Source: CAD feature listing. Evaluate the final solid. Frame: model axes, mm. Give positions to 0.01 mm unless a question says otherwise; leave off trailing zeros. Loops run counter-clockwise (first coordinate to the right, second up) from the corner with the lowest first, then second, coordinate; pieces in that order, holes last. Notation, with made-up numbers: (24.25, -12.5) - (43.25, -12.5) arc R24 ccw to (43.25, 19.5) - close; hole circle Ø7 at (66, 75). An arc over 180 degrees is marked (long way). Write each question's results on one line, items separated by ' | '. Start each with the question number.
(1) Cut plane B-B on y = 13.5. Return the cut outline in (x, z), then the cut area to 3 significant figures.
(2) Material intervals for line 1 along Z through (x, y) = (0.05, 14.75); line 2 along Y through (x, z) = (1.35, -2); line 3 along X through (y, z) = (1.5, -0.5), sorted ascending. Write a range as [from, to].
(3) Pull-direction query (X, two-part tool) for faces 1 (the flat face through (0, 21.7, 0)), 2 (the cylindrical face through (-1.5, 10.01, -0.07)), 3 (the flat face through (0, 0, 0)); classes: pulls with the +X half, pulls with the -X half, needs draft (parallel to the pull), parting line crosses it, or undercut.
(4) Contact query for flat-ended pins moving along their axis: pin 1 (2 mm diameter, centred on y = 15.5, z = 0, fed in from +X); pin 2 (2 mm diameter, centred on x = 1, y = 13.5, fed in from -Z). Output: stop coordinate, or through.
from build123d import *

# Parameters (mm, degrees)
SKETCH1_R           = 1.5
BOSS_EXTRUDE1_DEPTH = 22
SKETCH2_R           = 2.6
BOSS_EXTRUDE2_DEPTH = 1.7
BOSS_EXTRUDE2_TAPER = 32
SKETCH3_W           = 0.5
SKETCH3_H           = 1.758378485
SKETCH3_H_2         = 1.741621515
SKETCH3_W_2         = 1.734727157
SKETCH3_H_3         = 0.5
SKETCH3_W_3         = 1.765272843
CUT_EXTRUDE1_DEPTH  = 0.3


with BuildPart() as part:
    # Sketch1 → Boss-Extrude1 (new body)
    with BuildSketch(Plane(origin=(0, 0, 0), x_dir=(1, 0, 0), z_dir=(0, 1, 0))):
        Circle(SKETCH1_R)
    extrude(amount=BOSS_EXTRUDE1_DEPTH)

    # Sketch2 → Boss-Extrude2 (add)
    with BuildSketch(Plane(origin=(0, 22, 0), x_dir=(1, 0, 0), z_dir=(0, 1, 0))):
        Circle(SKETCH2_R)
    extrude(amount=-BOSS_EXTRUDE2_DEPTH, taper=BOSS_EXTRUDE2_TAPER)

    # Sketch3 → Cut-Extrude1 (cut)
    with BuildSketch(Plane(origin=(0, 22, 0), x_dir=(1, 0, 0), z_dir=(0, 1, 0))):
        with Locations((-0.015272843, 1.120810757)):
            Rectangle(SKETCH3_W, SKETCH3_H)
        with Locations((-0.015272843, -1.129189243)):
            Rectangle(SKETCH3_W, SKETCH3_H_2)
        with Locations((-1.132636421, -0.008378485)):
            Rectangle(SKETCH3_W_2, SKETCH3_H_3)
        with Locations((1.117363579, -0.008378485)):
            Rectangle(SKETCH3_W_3, SKETCH3_H_3)
        with Locations((-0.015272843, -0.008378485)):
            Rectangle(SKETCH3_W, SKETCH3_H_3)
    extrude(amount=-CUT_EXTRUDE1_DEPTH, mode=Mode.SUBTRACT)


solid = part.part
Ans:
1) outline: circle Ø3 at (0, 0) | area: 7.07 mm^2
2) line 1: [-1.5, 1.5] | line 2: [21.7, 22] | line 3: [-1.41, 1.41]
3) face 1: undercut | face 2: parting line crosses it | face 3: needs draft
4) pin 1: x = 1.5 | pin 2: z = -1.5
